Read the model definition and answer for the solid it produces. Units are mm, in the model's axes. A direction names the side the tool comes from. Round coordinates to 2 decimals unless told otherwise and drop trailing zeros. Order: outer loops, then holes, each group sorted by start corner. A loop starts at its lowest first (then second) coordinate and runs counter-clockwise, first axis right, second up. Notation, with made-up numbers: (37.5, 43.25) -> (55.5, 43.25) arc R10 cw to (55.5, 57.25) -> close; hole circle Ø10 at (83, -11). An arc over 180 degrees is marked (long way). One line per item, written item: value. Start each with the question number.
1. Section B-B (y = -17) is taken. Give the vertices of the cut face in (x, z) (3 decimals), then the cut area to 3 significant figures.
2. Section C-C (y = 22) is taken. Give the vertices of the cut face in (x, z) (3 decimals).
3. Section A-A (z = 1.3) is taken. State how many separate pieces and enclosed holes the cut face has, then the cut area to 3 significant figures.
4. The mould has two halves that part along X. Classify faces 6 (the face through (-12.7, -37, 2)), 7 (the face through (7.942, -18.841, 1.565)), 8 (the face through (25.4, -29, 2)), 9 (the face through (-19, -38.1, 2)): released by +X, released by -X, zero draft, split by the parting line, or undercut.
5. Section D-D (x = 4) is taken. Give the vertices of the cut face in (y, z) (3 decimals), then the cut area to 3 significant figures.
6. For faces 1 (the face through (9.19, 22.27, 1.57)), 2 (the face through (0, -34.925, 2)), 3 (the face through (-24, -19.05, 2)), 4 (the face through (0, 34.925, 2)), 5 (the face through (24, -19.05, 2)), determine the directions among +Z, -Z, +X, -X, +Y, -Y from which every point of the face is accessible in a straight line to the end or side of a thin tool.
7. Flat-ended cylindrical pins translate along their axes: pin 1 Ø1.6 at (x, z) = (-2.5, 2) entering from +Y (3 decimals); pin 2 Ø1 at (x, z) = (-1.5, 1.5) entering from -Y (3 decimals). Find the tip coordinate at first contact, or state that the pin passes through.
8. Consider line 1 (Y direction, x = -12, z = 2.7) (3 decimals); line 2 (X direction, y = -13.5, z = 0.65) (3 decimals); line 3 (X direction, y = -18.5, z = 1.8) (3 decimals). Determine where each line is inside the solid, lowest interval first.
from build123d import *

# Parameters (mm, degrees)
F0_R     = 4.7625
F1_DEPTH = 3.175


with BuildPart() as f1:
    # F0 (on Top) → F1 (new body)
    with BuildSketch(Plane.XY):
        Polygon((25.4, 19.05), (25.4, 38.1), (12.7, 38.1), (12.7, 34.925), (-12.7, 34.925), (-12.7, 38.1), (-25.4, 38.1), (-25.4, 19.05), (-22.225, 19.05), (-22.225, -19.05), (-25.4, -19.05), (-25.4, -38.1), (-12.7, -38.1), (-12.7, -34.925), (12.7, -34.925), (12.7, -38.1), (25.4, -38.1), (25.4, -19.05), (22.225, -19.05), (22.225, 19.05), align=None)
        with Locations((12.7, -19.05)):
            Circle(F0_R, mode=Mode.SUBTRACT)
        with Locations((12.7, 19.05)):
            Circle(F0_R, mode=Mode.SUBTRACT)
    extrude(amount=F1_DEPTH)


solid = f1.part
Answer:
1. outline: (-22.225, 0) -> (8.401, 0) -> (8.401, 3.175) -> (-22.225, 3.175) -> close; (16.999, 0) -> (22.225, 0) -> (22.225, 3.175) -> (16.999, 3.175) -> close
1. area: 114 mm^2
2. outline: (-25.4, 0) -> (8.961, 0) -> (8.961, 3.175) -> (-25.4, 3.175) -> close; (16.439, 0) -> (25.4, 0) -> (25.4, 3.175) -> (16.439, 3.175) -> close
3. separate pieces: 1
3. enclosed holes: 2
3. area: 3,330 mm^2
4. face 6: undercut
4. face 7: undercut
4. face 8: released by +X
4. face 9: zero draft
5. outline: (-34.925, 0) -> (34.925, 0) -> (34.925, 3.175) -> (-34.925, 3.175) -> close
5. area: 222 mm^2
6. face 1: +Z, -Z
6. face 2: +Z, -Z, -Y
6. face 3: +Z, -Z, -X
6. face 4: +Z, -Z, +Y
6. face 5: +Z, -Z, +X
7. pin 1: y = 34.925
7. pin 2: y = -34.925
8. line 1: -34.925 to 34.925
8. line 2: -22.225 to 22.225
8. line 3: -22.225 to 7.969, 17.431 to 22.225
